Here's how the part is built. I have some questions about the finished solid (model axes, mm). Round coordinates to 2 decimals unless told otherwise and drop trailing zeros. Write each loop counter-clockwise with the first axis right and the second up, starting at its lowest first coordinate (ties: lowest second). Pieces come first, ordered by that corner, then holes. Notation, with made-up numbers: (-16, -19.5) -> (9, -19.5) arc R28 cw to (9, 0.5) -> close; hole circle Ø9 at (73, 54). An arc over 180 degrees is marked (long way). Answer in a Markdown table with one row per item.
from build123d import *

# Parameters (mm, degrees)
F2_DEPTH = 3.175


with BuildPart() as f2:
    # F1 (on offset) → F2 (new body)
    with BuildSketch(Plane.YZ.offset(142.875)):
        Polygon((225.425, -19.05), (225.425, 44.45), (-225.425, 44.45), (-225.425, -19.05), (-200.025, -44.45), (200.025, -44.45), align=None)
    extrude(amount=F2_DEPTH)


solid = f2.part
1) I want a section at A-A, the plane x = 144.2. List the corners of the cut face in (y, z) for me (3 decimals), and give its area (3 significant figures).
Response:
| item | result |
|---|---|
| outline | (-225.425, -19.05) -> (-200.025, -44.45) -> (200.025, -44.45) -> (225.425, -19.05) -> (225.425, 44.45) -> (-225.425, 44.45) -> close |
| area | 39,400 mm^2 |
2) I need wall thicknesses on line 1 (Y direction, x = 145.65, z = -34) (3 decimals); line 2 (Y direction, x = 143.25, z = -37) (3 decimals). Which ranges of each line are inside material? Lowest first, please. Write a range as [from, to].
Response:
| item | result |
|---|---|
| line 1 | y = [-210.475, 210.475] |
| line 2 | y = [-207.475, 207.475] |
3) I want a section at B-B, the plane z = -29. List the corners of the cut face in (x, y) for me (3 decimals).
Response:
| item | result |
|---|---|
| outline | (142.875, -215.475) -> (146.05, -215.475) -> (146.05, 215.475) -> (142.875, 215.475) -> close |
